Part model, mm, in its own coordinate system. Round coordinates to 2 decimals unless told otherwise and drop trailing zeros. Order: outer loops, then holes, each group sorted by start corner. A loop starts at its lowest first (then second) coordinate and runs counter-clockwise, first axis right, second up. Notation, with made-up numbers: (-22, 15) - (-3, 15) arc R20 cw to (-3, 32) - close; hole circle Ø3 at (11.5, -17). An arc over 180 degrees is marked (long way). Answer as a JSON object with one key per item and string values.
```python
from build123d import *

# Parameters (mm, degrees)
SKETCH_1_W          = 100
SKETCH_1_H          = 80
SKETCH_1_R          = 1.35
EXTRUDE_1_DEPTH     = 2
SKETCH_2_W          = 8
SKETCH_2_H          = 80
CUT_EXTRUDE_1_DEPTH = 5
SKETCH_3_R          = 1.6
CUT_EXTRUDE_2_DEPTH = 5
SKETCH_4_W          = 30
SKETCH_4_H          = 80
EXTRUDE_2_DEPTH     = 2
SKETCH_5_R          = 1.6
CUT_EXTRUDE_3_DEPTH = 2
SKETCH_6_W          = 43.75
SKETCH_6_H          = 3
SKETCH_6_W_2        = 7
CUT_EXTRUDE_4_DEPTH = 10
SKETCH_8_R          = 1.6
CUT_EXTRUDE_5_DEPTH = 10
SKETCH_7_W          = 64
SKETCH_7_H          = 28
SKETCH_7_W_2        = 32.75
CUT_EXTRUDE_6_DEPTH = 10
EXTRUDE_1_2_DEPTH   = 2
FILLET_1_R          = 2
FILLET_2_R          = 1.5


with BuildPart() as part:
    # 草图1 → Extrude 1 (new body)
    with BuildSketch(Plane(origin=(0, 0, 0), x_dir=(1, 0, 0), z_dir=(0, 1, 0))):
        Rectangle(SKETCH_1_W, SKETCH_1_H)
        with Locations(Location((18, -18, 0), (0, 0, 270))):
            Circle(SKETCH_1_R, mode=Mode.SUBTRACT)
        with Locations(Location((-18, -18, 0), (0, 0, 270))):
            Circle(SKETCH_1_R, mode=Mode.SUBTRACT)
        with Locations(Location((-18, 18, 0), (0, 0, 270))):
            Circle(SKETCH_1_R, mode=Mode.SUBTRACT)
        with Locations(Location((18, 18, 0), (0, 0, 270))):
            Circle(SKETCH_1_R, mode=Mode.SUBTRACT)
    extrude(amount=EXTRUDE_1_DEPTH)

    # 草图2 → 切除-拉伸1 (cut)
    with BuildSketch(Plane(origin=(0, 2, 0), x_dir=(1, 0, 0), z_dir=(0, 1, 0))):
        with Locations((-46, 0)):
            Rectangle(SKETCH_2_W, SKETCH_2_H)
    extrude(amount=-CUT_EXTRUDE_1_DEPTH, mode=Mode.SUBTRACT)

    # 草图3 → 切除-拉伸2 (cut)
    with BuildSketch(Plane(origin=(0, 2, 0), x_dir=(1, 0, 0), z_dir=(0, 1, 0))):
        with Locations(Location((-39.25, -22, 0), (0, 0, 270))):
            Circle(SKETCH_3_R)
        with Locations(Location((-39.25, -2, 0), (0, 0, 270))):
            Circle(SKETCH_3_R)
        with Locations(Location((39.25, -22, 0), (0, 0, 270))):
            Circle(SKETCH_3_R)
        with Locations(Location((39.25, -2, 0), (0, 0, 270))):
            Circle(SKETCH_3_R)
    extrude(amount=-CUT_EXTRUDE_2_DEPTH, mode=Mode.SUBTRACT)

    # 草图4 → 凸台-拉伸2 (add)
    with BuildSketch(Plane(origin=(0, 2, 0), x_dir=(1, 0, 0), z_dir=(0, 1, 0))):
        with Locations((65, 0)):
            Rectangle(SKETCH_4_W, SKETCH_4_H)
    extrude(amount=-EXTRUDE_2_DEPTH)

    # 草图5 → 切除-拉伸3 (cut)
    with BuildSketch(Plane(origin=(0, 2, 0), x_dir=(1, 0, 0), z_dir=(0, 1, 0))):
        with Locations(Location((34.5, -18, 0), (0, 0, 270))):
            Circle(SKETCH_5_R)
        with Locations(Location((70.5, -18, 0), (0, 0, 270))):
            Circle(SKETCH_5_R)
        with Locations(Location((70.5, 18, 0), (0, 0, 270))):
            Circle(SKETCH_5_R)
        with Locations(Location((34.5, 18, 0), (0, 0, 270))):
            Circle(SKETCH_5_R)
    extrude(amount=-CUT_EXTRUDE_3_DEPTH, mode=Mode.SUBTRACT)

    # 草图6 → 切除-拉伸4 (cut)
    with BuildSketch(Plane(origin=(0, 2, 0), x_dir=(1, 0, 0), z_dir=(0, 1, 0))):
        with Locations((58.125, -38.5)):
            Rectangle(SKETCH_6_W, SKETCH_6_H)
        with Locations((-38.5, -38.5)):
            Rectangle(SKETCH_6_W_2, SKETCH_6_H)
    extrude(amount=-CUT_EXTRUDE_4_DEPTH, mode=Mode.SUBTRACT)

    # 草图8 → 切除-拉伸5 (cut)
    with BuildSketch(Plane(origin=(0, 2, 0), x_dir=(1, 0, 0), z_dir=(0, 1, 0))):
        with Locations(Location((77.75, -33, 0), (0, 0, 270))):
            Circle(SKETCH_8_R)
        with Locations(Location((77.75, 35, 0), (0, 0, 270))):
            Circle(SKETCH_8_R)
        with Locations(Location((-33.25, 35, 0), (0, 0, 270))):
            Circle(SKETCH_8_R)
    extrude(amount=-CUT_EXTRUDE_5_DEPTH, mode=Mode.SUBTRACT)

    # 草图7 → 切除-拉伸6 (cut)
    with BuildSketch(Plane(origin=(0, 2, 0), x_dir=(1, 0, 0), z_dir=(0, 1, 0))):
        with BuildLine():
            Line((-25, -22), (25, -22))
            ThreePointArc((25, -22), (32, -29), (25, -36))
            Line((25, -36), (-25, -36))
            ThreePointArc((-25, -36), (-32, -29), (-25, -22))
        make_face()
        with BuildLine():
            Line((45.25, -25), (69, -25))
            ThreePointArc((69, -25), (73, -29), (69, -33))
            Line((69, -33), (45.25, -33))
            ThreePointArc((45.25, -33), (41.25, -29), (45.25, -25))
        make_face()
        Rectangle(SKETCH_7_W, SKETCH_7_H)
        with Locations((59.625, 0)):
            Rectangle(SKETCH_7_W_2, SKETCH_7_H)
        with BuildLine():
            Line((-18.25, 36), (62.75, 36))
            ThreePointArc((62.75, 36), (70.25, 28.5), (62.75, 21))
            Line((62.75, 21), (-18.25, 21))
            ThreePointArc((-18.25, 21), (-25.75, 28.5), (-18.25, 36))
        make_face()
    extrude(amount=-CUT_EXTRUDE_6_DEPTH, mode=Mode.SUBTRACT)

    # 草图9 → Extrude 1 2 (add)
    with BuildSketch(Plane(origin=(0, 2, 0), x_dir=(1, 0, 0), z_dir=(0, 1, 0))):
        Polygon((32.601228251, -12.625763998), (-31.398771749, 15.374236002), (-32.601228251, 12.625763998), (31.398771749, -15.374236002), align=None)
        Polygon((-31.398771749, -15.374236002), (32.601228251, 12.625763998), (31.398771749, 15.374236002), (-32.601228251, -12.625763998), align=None)
        Polygon((42.275247173, 12.859887319), (75.025247173, -15.140112681), (76.974752827, -12.859887319), (44.224752827, 15.140112681), align=None)
        Polygon((44.224752827, -15.140112681), (76.974752827, 12.859887319), (75.025247173, 15.140112681), (42.275247173, -12.859887319), align=None)
    extrude(amount=-EXTRUDE_1_2_DEPTH)

    # 圆角1
    fillet_1_edges = [part.edges().sort_by_distance(p)[0] for p in [
        (28.257660886, 1, -14),
        (-28.257660886, 1, -14),
        (-32, 1, 12.362726638),
        (-32, 1, -12.362726638),
        (-28.257660886, 1, 14),
        (28.257660886, 1, 14),
        (32, 1, -12.362726638),
        (32, 1, 12.362726638),
        (3.742339114, 1, 0),
        (0, 1, 1.637273362),
        (-3.742339114, 1, 0),
        (0, 1, -1.637273362),
        (45.558277481, 1, 14),
        (73.691722519, 1, 14),
        (76, 1, -12.026510856),
        (76, 1, 12.026510856),
        (73.691722519, 1, -14),
        (45.558277481, 1, -14),
        (43.25, 1, 12.026510856),
        (43.25, 1, -12.026510856),
        (57.316722519, 1, 0),
        (59.625, 1, -1.973489144),
        (61.933277481, 1, 0),
        (59.625, 1, 1.973489144),
    ]]
    fillet(fillet_1_edges, radius=FILLET_1_R)

    # 圆角2
    fillet_2_edges = [part.edges().sort_by_distance(p)[0] for p in [
        (80, 1, 37),
        (80, 1, -40),
        (-42, 1, -40),
        (-42, 1, 37),
        (-35, 1, 37),
        (-35, 1, 40),
        (36.25, 1, 37),
        (36.25, 1, 40),
    ]]
    fillet(fillet_2_edges, radius=FILLET_2_R - 0.0001)  # a hair under: the kernel refuses the full size


solid = part.part
```
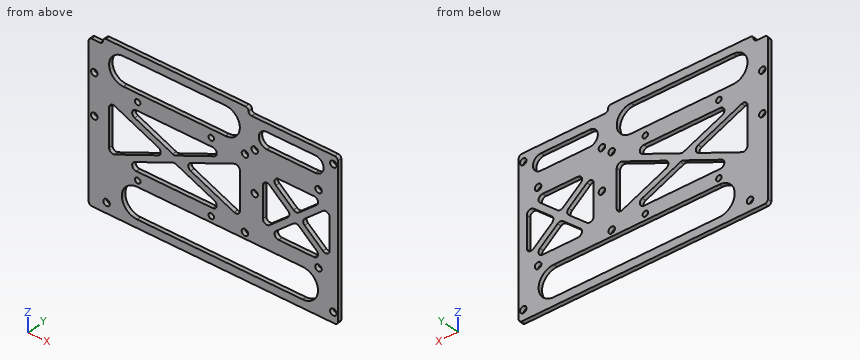
Item 1: Cut at B-B (z = -26). Write the cut outline in (x, y).
Taken from the geometry:
{"outline": "(-42, 0) - (-25.32, 0) - (-25.32, 2) - (-42, 2) - close; (69.82, 0) - (80, 0) - (80, 2) - (69.82, 2) - close"}
Item 2: Cut at D-D (y = 0.8). State how many separate pieces and enclosed holes the cut face has, plus the area to 3 significant figures.
Taken from the geometry:
{"separate pieces": "1", "enclosed holes": "26", "area": "5,050 mm2"}
Item 3: Probe L1, parallel to X at y = 0.9, z = 18; L2, parallel to X at y = 1.1, z = 29; L3, parallel to Z at x = 39, y = 1.35. List the from-to ranges inside material, lowest first. Write a range as from..to.
Taken from the geometry:
{"L1": "-42..-19.35, -16.65..16.65, 19.35..32.9, 36.1..68.9, 72.1..80", "L2": "-42..-32, 32..41.25, 73..80", "L3": "-40..-36, -21..0.42, 3.58..20.42, 23.58..37"}
Item 4: Cut at A-A (x = -39.25). Write the cut outline in (y, z), plus the area to 3 significant figures.
Taken from the geometry:
{"outline": "(0, -40) - (2, -40) - (2, 0.4) - (0, 0.4) - close; (0, 3.6) - (2, 3.6) - (2, 20.4) - (0, 20.4) - close; (0, 23.6) - (2, 23.6) - (2, 37) - (0, 37) - close", "area": "141 mm2"}
Item 5: Cut at C-C (x = -15). Write the cut outline in (y, z), plus the area to 3 significant figures.
Taken from the geometry:
{"outline": "(0, -40) - (2, -40) - (2, -36) - (0, -36) - close; (0, -21) - (2, -21) - (2, -14) - (0, -14) - close; (0, -8.2) - (2, -8.2) - (2, -4.93) - (0, -4.93) - close; (0, 4.93) - (2, 4.93) - (2, 8.2) - (0, 8.2) - close; (0, 14) - (2, 14) - (2, 22) - (0, 22) - close; (0, 36) - (2, 36) - (2, 40) - (0, 40) - close", "area": "59.1 mm2"}
Item 6: Drop a flat-ended pin along its axis: P1, Ø0.6, axis at x = 62.5, y = 1.5, coming from the +Z side. Give the stop position or say it passes through.
Taken from the geometry:
{"P1": "z = 37"}
